from build123d import *

# Parameters (mm, degrees)
SKETCH1_W           = 7
SKETCH1_H           = 6
BOSS_EXTRUDE2_DEPTH = 8
CUT_EXTRUDE2_DEPTH  = 7
CUT_EXTRUDE3_DEPTH  = 4
CUT_EXTRUDE4_DEPTH  = 2
CUT_EXTRUDE5_DEPTH  = 1
SKETCH10_W          = 2
SKETCH10_H          = 3.605551276
CUT_EXTRUDE6_DEPTH  = 3.496150883


with BuildPart() as part:
    # Sketch1 → Boss-Extrude2 (new body)
    with BuildSketch(Plane.XY):
        Rectangle(SKETCH1_W, SKETCH1_H)
    extrude(amount=BOSS_EXTRUDE2_DEPTH)

    # Sketch4 → Cut-Extrude2 (cut, through all)
    with BuildSketch(Plane(origin=(0, 3, 0), x_dir=(1, 0, 0), z_dir=(0, 1, 0))):
        Polygon((3.5, -2), (1.5, -2), (1.5, -4), (-0.5, -4), (-0.5, -7), (-1.5, -8), (3.5, -8), align=None)
    extrude(amount=-CUT_EXTRUDE2_DEPTH, mode=Mode.SUBTRACT)

    # Sketch5 → Cut-Extrude3 (cut)
    with BuildSketch(Plane(origin=(0, 3, 0), x_dir=(1, 0, 0), z_dir=(0, 1, 0))):
        Polygon((1.5, -4), (1.5, -2), (-1.5, -2), (-1.5, -7), (-3.5, -7), (-3.5, -8), (-1.5, -8), (-0.5, -7), (-0.5, -4), align=None)
    extrude(amount=-CUT_EXTRUDE3_DEPTH, mode=Mode.SUBTRACT)

    # Sketch6 → Cut-Extrude4 (cut)
    with BuildSketch(Plane(origin=(0, 0, 0), x_dir=(-1, 0, 0), z_dir=(0, 0, -1))):
        Polygon((-3.5, -1), (-0.5, 1), (-0.5, 3), (-3.5, 3), align=None)
    extrude(amount=-CUT_EXTRUDE4_DEPTH, mode=Mode.SUBTRACT)

    # Sketch7 → Cut-Extrude5 (cut)
    with BuildSketch(Plane(origin=(0, 3, 0), x_dir=(1, 0, 0), z_dir=(0, 1, 0))):
        Polygon((-0.5, -2), (-0.5, -1), (-2.5, -1), (-2.5, -6), (-1.5, -6), (-1.5, -2), align=None)
    extrude(amount=-CUT_EXTRUDE5_DEPTH, mode=Mode.SUBTRACT)

    # Sketch10 → Cut-Extrude6 (cut, through all)
    with BuildSketch(Plane(origin=(0, 3.230769231, 4.846153846), x_dir=(-1, 0, 0), z_dir=(0, -0.554700196, -0.832050294))):
        with Locations((2.5, -2.080125736)):
            Rectangle(SKETCH10_W, SKETCH10_H)
    extrude(amount=-CUT_EXTRUDE6_DEPTH, mode=Mode.SUBTRACT)


solid = part.part
Read the model definition and answer for the solid it produces. Units are mm, in the model's axes. A direction names the side the tool comes from. Give positions to 0.01 mm unless a question says otherwise; leave off trailing zeros. Write each loop counter-clockwise with the first axis right and the second up, starting at its lowest first coordinate (ties: lowest second). Pieces come first, ordered by that corner, then holes. Notation, with made-up numbers: M -20,87.25 L 20,87.25 A18 cw 20,101.25 Z; hole C 64.5,85 d9. An arc over 180 degrees is marked long. One line per item, written item: value. Start each with the question number.
(1) Find the intervals of material crossed by line 1 (Y direction, x = 0.75, z = 3); line 2 (X direction, y = 0.5, z = 6.25); line 3 (Z direction, x = 3, y = -1.75), in increasing order.
(2) A tool of negligible diameter and unlimited length cuts with its end or side. For faces 4 (the flat face through (-1.5, 2.5, 1)), 5 (the flat face through (-2.5, -0.5, 7)), 6 (the flat face through (1, -2, 4)), 7 (the flat face through (-1.5, 1, 4)), 8 (the flat face through (-1, -3, 3)), from which of +Z, -Z, +X, -X, +Y, -Y can it reach the whole face along a straight path? Write none if from no direction.
(3) Find section B-B (x = -2.75). Determine the outline of the cut face in (y, z), plus the area to 3 significant figures.
(4) Determine the mould class of faces 1 (the flat face through (2, 0, 1)), 2 (the flat face through (-2.5, 2.5, 3.3)), 3 (the flat face through (-1, -1, 4)) for opening direction X: pulls with the +X half, pulls with the -X half, needs draft (parallel to the pull), parting line crosses it, or undercut.
(5) Find section A-A (z = 2.5). Determine the outline of the cut face in (x, y), plus the area to 3 significant figures.
(6) Flat-ended cylindrical pins translate along their axes: pin 1 Ø0.8 at (y, z) = (2.5, 3) entering from +X; pin 2 Ø1.5 at (y, z) = (1, 1) entering from +X (3 decimals); pin 3 Ø1 at (y, z) = (-2.5, 5) entering from +X. Find the tip coordinate at first contact, or state that the pin passes through.
(7) Find section D-D (y = -1.5). Determine the outline of the cut face in (x, z), plus the area to 3 significant figures.
(8) Find section C-C (y = 1.5). Determine the outline of the cut face in (x, z), plus the area to 3 significant figures.
Results below:
1. line 1: y = -3 to -1
1. line 2: x = -3.5 to -1.5
1. line 3: z = 0 to 2
2. face 4: +Z, +Y
2. face 5: +Z, +X, -X, +Y
2. face 6: +Z, +X, +Y, -Y
2. face 7: +Z, +X, +Y
2. face 8: +Z, -Z, +X, -X, -Y
3. outline: M -3,0 L 3,0 L 3,5 L 0,7 L -1,7 L -1,8 L -3,8 Z
3. area: 41.0 mm^2
4. face 1: pulls with the +X half
4. face 2: undercut
4. face 3: needs draft
5. outline: M -3.5,-3 L 1.5,-3 L 1.5,-1 L -1.5,-1 L -1.5,2 L -2.5,2 L -2.5,3 L -3.5,3 Z
5. area: 17.0 mm^2
6. pin 1: stops at x = -2.5
6. pin 2: stops at x = 1.625
6. pin 3: stops at x = -0.5
7. outline: M -3.5,0 L 3.5,0 L 3.5,2 L 1.5,2 L 1.5,4 L -0.5,4 L -0.5,7 L -1.5,8 L -3.5,8 Z
7. area: 35.5 mm^2
8. outline: M -3.5,0 L 0.5,0 L 0.5,2 L -1.5,2 L -1.5,6 L -3.5,6 Z
8. area: 16.0 mm^2
